from build123d import *

# Parameters (mm, degrees)
F0_W       = 85
F0_H       = 85
F1_DEPTH   = 3
F2_W       = 13.4
F2_H       = 13.4
F3_DEPTH   = 25
F5_DEPTH   = 15
F6_SIZE2   = 14.99999
F6_SIZE    = 9.99999
F6_2_SIZE2 = 14.99999
F6_2_SIZE  = 9.99999
F6_3_SIZE2 = 14.99999
F6_3_SIZE  = 9.99999
F6_4_SIZE2 = 14.99999
F6_4_SIZE  = 9.99999
F7_SIZE2   = 9.99999
F7_SIZE    = 14.99999
F7_2_SIZE2 = 9.99999
F7_2_SIZE  = 14.99999
F7_3_SIZE2 = 9.99999
F7_3_SIZE  = 14.99999
F7_4_SIZE2 = 9.99999
F7_4_SIZE  = 14.99999
F7_5_SIZE2 = 9.99999
F7_5_SIZE  = 14.99999
F9_DEPTH   = 68.601
F11_DEPTH  = 68.601


# Not quite as in the source:
# - a fillet or chamfer is up to 0.001 mm smaller than in the source, because OpenCascade refuses the exact size
# - a feature names something its author has since deleted; it is built from what else it names


with BuildPart() as f1:
    # F0 (on Top) → F1 (new body)
    with BuildSketch(Plane.XY):
        Rectangle(F0_W, F0_H)
    extrude(amount=F1_DEPTH)

    # F2 (on face) → F3 (cut)
    with BuildSketch(Plane.XY.offset(3)):
        with Locations((-32.8, 16.4)):
            Rectangle(F2_W, F2_H)
        with Locations((-32.8, 0)):
            Rectangle(F2_W, F2_H)
        with Locations((-32.8, -16.4)):
            Rectangle(F2_W, F2_H)
        with Locations((-32.8, -32.8)):
            Rectangle(F2_W, F2_H)
        with Locations((-16.4, 32.8)):
            Rectangle(F2_W, F2_H)
        with Locations((-16.4, 16.4)):
            Rectangle(F2_W, F2_H)
        with Locations((-16.4, 0)):
            Rectangle(F2_W, F2_H)
        with Locations((-16.4, -16.4)):
            Rectangle(F2_W, F2_H)
        with Locations((-16.4, -32.8)):
            Rectangle(F2_W, F2_H)
        with Locations((0, 32.8)):
            Rectangle(F2_W, F2_H)
        with Locations((0, 16.4)):
            Rectangle(F2_W, F2_H)
        Rectangle(F2_W, F2_H)
        with Locations((0, -16.4)):
            Rectangle(F2_W, F2_H)
        with Locations((0, -32.8)):
            Rectangle(F2_W, F2_H)
        with Locations((16.4, 32.8)):
            Rectangle(F2_W, F2_H)
        with Locations((16.4, 16.4)):
            Rectangle(F2_W, F2_H)
        with Locations((16.4, 0)):
            Rectangle(F2_W, F2_H)
        with Locations((16.4, -16.4)):
            Rectangle(F2_W, F2_H)
        with Locations((16.4, -32.8)):
            Rectangle(F2_W, F2_H)
        with Locations((32.8, 32.8)):
            Rectangle(F2_W, F2_H)
        with Locations((32.8, 16.4)):
            Rectangle(F2_W, F2_H)
        with Locations((32.8, 0)):
            Rectangle(F2_W, F2_H)
        with Locations((32.8, -16.4)):
            Rectangle(F2_W, F2_H)
        with Locations((32.8, -32.8)):
            Rectangle(F2_W, F2_H)
        with Locations((-32.8, 32.8)):
            Rectangle(F2_W, F2_H)
    extrude(amount=-F3_DEPTH, mode=Mode.SUBTRACT)

    # F4 (on face) → F5 (join)
    with BuildSketch(Plane.XY.offset(3)):
        Polygon((-23.1, -9.7), (-26.1, -9.7), (-26.1, -23.1), (-39.5, -23.1), (-39.5, -26.1), (-26.1, -26.1), (-26.1, -39.5), (-23.1, -39.5), (-23.1, -26.1), (-9.7, -26.1), (-9.7, -23.1), (-23.1, -23.1), align=None)
        Polygon((-9.7, 23.1), (-9.7, 26.1), (-23.1, 26.1), (-23.1, 39.5), (-26.1, 39.5), (-26.1, 26.1), (-39.5, 26.1), (-39.5, 23.1), (-26.1, 23.1), (-26.1, 9.7), (-23.1, 9.7), (-23.1, 23.1), align=None)
        Polygon((26.1, 26.1), (26.1, 39.5), (23.1, 39.5), (23.1, 26.1), (9.7, 26.1), (9.7, 23.1), (23.1, 23.1), (23.1, 9.7), (26.1, 9.7), (26.1, 23.1), (39.5, 23.1), (39.5, 26.1), align=None)
        Polygon((26.1, -23.1), (26.1, -9.7), (23.1, -9.7), (23.1, -23.1), (9.7, -23.1), (9.7, -26.1), (23.1, -26.1), (23.1, -39.5), (26.1, -39.5), (26.1, -26.1), (39.5, -26.1), (39.5, -23.1), align=None)
    extrude(amount=F5_DEPTH)

    # F6 (size 10 and 15 in the source; OpenCascade refuses exactly that, so slightly less here)
    f6_edges = [f1.edges().sort_by_distance(p)[0] for p in [
        (-39.5, -24.6, 18),
        (-24.6, -9.7, 18),
        (-9.7, -24.6, 18),
        (-24.6, -39.5, 18),
    ]]
    f6_side = f1.faces().sort_by_distance((-24.6, -24.6, 18))[0]
    chamfer(f6_edges, length=F6_SIZE, length2=F6_SIZE2, reference=f6_side)

    # F6#2 (size 10 and 15 in the source; OpenCascade refuses exactly that, so slightly less here)
    f6_2_edges = [f1.edges().sort_by_distance(p)[0] for p in [
        (-39.5, 24.6, 18),
        (-24.6, 39.5, 18),
    ]]
    f6_2_side = f1.faces().sort_by_distance((-24.6, 24.6, 18))[0]
    chamfer(f6_2_edges, length=F6_2_SIZE, length2=F6_2_SIZE2, reference=f6_2_side)

    # F6#3 (size 10 and 15 in the source; OpenCascade refuses exactly that, so slightly less here)
    f6_3_edges = [f1.edges().sort_by_distance(p)[0] for p in [
        (9.7, 24.6, 18),
        (24.6, 39.5, 18),
    ]]
    f6_3_side = f1.faces().sort_by_distance((24.6, 24.6, 18))[0]
    chamfer(f6_3_edges, length=F6_3_SIZE, length2=F6_3_SIZE2, reference=f6_3_side)

    # F6#4 (size 10 and 15 in the source; OpenCascade refuses exactly that, so slightly less here)
    f6_4_edges = [f1.edges().sort_by_distance(p)[0] for p in [
        (24.6, -9.7, 18),
        (9.7, -24.6, 18),
        (39.5, -24.6, 18),
    ]]
    f6_4_side = f1.faces().sort_by_distance((24.6, -24.6, 18))[0]
    chamfer(f6_4_edges, length=F6_4_SIZE, length2=F6_4_SIZE2, reference=f6_4_side)

    # F7 (size 15 and 10 in the source; OpenCascade refuses exactly that, so slightly less here)
    f7_edges = [f1.edges().sort_by_distance(p)[0] for p in [
        (-9.7, 24.6, 18),
    ]]
    f7_side = f1.faces().sort_by_distance((-9.7, 24.6, 10.5))[0]
    chamfer(f7_edges, length=F7_SIZE, length2=F7_SIZE2, reference=f7_side)

    # F7#2 (size 15 and 10 in the source; OpenCascade refuses exactly that, so slightly less here)
    f7_2_edges = [f1.edges().sort_by_distance(p)[0] for p in [
        (-24.6, 9.7, 18),
    ]]
    f7_2_side = f1.faces().sort_by_distance((-24.6, 9.7, 10.5))[0]
    chamfer(f7_2_edges, length=F7_2_SIZE, length2=F7_2_SIZE2, reference=f7_2_side)

    # F7#3 (size 15 and 10 in the source; OpenCascade refuses exactly that, so slightly less here)
    f7_3_edges = [f1.edges().sort_by_distance(p)[0] for p in [
        (24.6, 9.7, 18),
    ]]
    f7_3_side = f1.faces().sort_by_distance((24.6, 9.7, 10.5))[0]
    chamfer(f7_3_edges, length=F7_3_SIZE, length2=F7_3_SIZE2, reference=f7_3_side)

    # F7#4 (size 15 and 10 in the source; OpenCascade refuses exactly that, so slightly less here)
    f7_4_edges = [f1.edges().sort_by_distance(p)[0] for p in [
        (39.5, 24.6, 18),
    ]]
    f7_4_side = f1.faces().sort_by_distance((39.5, 24.6, 10.5))[0]
    chamfer(f7_4_edges, length=F7_4_SIZE, length2=F7_4_SIZE2, reference=f7_4_side)

    # F7#5 (size 15 and 10 in the source; OpenCascade refuses exactly that, so slightly less here)
    f7_5_edges = [f1.edges().sort_by_distance(p)[0] for p in [
        (24.6, -39.5, 18),
    ]]
    f7_5_side = f1.faces().sort_by_distance((24.6, -39.5, 10.5))[0]
    chamfer(f7_5_edges, length=F7_5_SIZE, length2=F7_5_SIZE2, reference=f7_5_side)

    # F8 (on face) → F9 (cut, through all)
    with BuildSketch(Plane.YZ.offset(26.1)):
        Polygon((-26.1, 17), (-26.5611153912, 17), (-35.8944487245, 3), (-26.1, 3), align=None)
        Polygon((-22.6388846088, 17), (-23.1, 17), (-23.1, 3), (-13.3055512755, 3), align=None)
        Polygon((23.1, 17), (22.6388846088, 17), (13.3055512755, 3), (23.1, 3), align=None)
        Polygon((26.5611153912, 17), (26.1, 17), (26.1, 3), (35.8944487245, 3), align=None)
    extrude(amount=-F9_DEPTH, mode=Mode.SUBTRACT)

    # F10 (on face) → F11 (cut, through all)
    with BuildSketch(Plane.XZ.offset(26.1)):
        Polygon((-26.1, 17), (-26.5611153912, 17), (-35.8944487245, 3), (-26.1, 3), align=None)
        Polygon((-22.6388846088, 17), (-23.1, 17), (-23.1, 3), (-13.3055512755, 3), align=None)
        Polygon((23.1, 17), (22.6388846088, 17), (13.3055512755, 3), (23.1, 3), align=None)
        Polygon((26.5611153912, 17), (26.1, 17), (26.1, 3), (35.8944487245, 3), align=None)
    extrude(amount=-F11_DEPTH, mode=Mode.SUBTRACT)


solid = f1.part
CAD build for the part. Positions are in the model's coordinates, mm. A direction names the side the tool comes from. Round coordinates to 2 decimals unless told otherwise and drop trailing zeros. Order: outer loops, then holes, each group sorted by start corner. A loop starts at its lowest first (then second) coordinate and runs counter-clockwise, first axis right, second up. Notation, with made-up numbers: (52.25, 5) -> (79.25, 5) arc R31 cw to (79.25, 32) -> close; hole circle Ø6 at (-38.75, 49.25). An arc over 180 degrees is marked (long way). Write item = value, one per line. Start each with the question number.
(1) Pin check, flat tips, straight feed: P1, Ø6.5, axis at y = 33, z = 12.5, coming from the -X side; P2, Ø2, axis at y = -33.5, z = 5.5, coming from the +X side; P3, Ø1, axis at x = 12, y = 21.5, coming from the -Z side; P4, Ø0.5, axis at x = -26.5, y = -24.5, coming from the -Z side. Stop position of each tip, or through.
(2) Cut at A-A, the plane y = -2.5. List the corners of the cut face in (x, z).
(3) Pull direction Y, two halves, no side cores. Call faces 5 (the flat face through (-23.1, 15, 7)), 6 (the flat face through (-26.1, 25, 10)): released by +Y, released by -Y, zero draft, split by the parting line, or undercut.
(4) Probe line 1 (Y direction, x = 19, z = 1.75); line 2 (Y direction, x = 38, z = 4.5). List the from-to ranges inside material, lowest first. Write a range as [from, to].
(5) Which spindle directions (+Z, -Z, +X, -X, +Y, -Y) get a long thin tool onto all of the face, cutting with end or side? Do faces 1 (the flat face through (-24.621, 14.77, 10.605)), 2 (the flat face through (33, 9.7, 2)), 3 (the flat face through (-25, -18, 3)), 4 (the flat face through (-18, 25, 3)). Say none if no direction does.
(6) Cut at B-B, the plane y = -31.5. State how many separate pieces and enclosed holes the cut face has, then the cut area to 4 significant figures.
Model answer:
q1.P1 = -26.1
q1.P2 = 26.1
q1.P3 = through
q1.P4 = 0
q2.outline = (-42.5, 0) -> (-39.5, 0) -> (-39.5, 3) -> (-42.5, 3) -> close; (-26.1, 0) -> (-23.1, 0) -> (-23.1, 3) -> (-26.1, 3) -> close; (-9.7, 0) -> (-6.7, 0) -> (-6.7, 3) -> (-9.7, 3) -> close; (6.7, 0) -> (9.7, 0) -> (9.7, 3) -> (6.7, 3) -> close; (23.1, 0) -> (26.1, 0) -> (26.1, 3) -> (23.1, 3) -> close; (39.5, 0) -> (42.5, 0) -> (42.5, 3) -> (39.5, 3) -> close
q3.face_5 = undercut
q3.face_6 = zero draft
q4.line_1 = [-42.5, -39.5], [-26.1, -23.1], [-9.7, -6.7], [6.7, 9.7], [23.1, 26.1], [39.5, 42.5]
q4.line_2 = [-26.1, -23.1], [23.1, 26.1]
q5.face_1 = +Z, +X, -X
q5.face_2 = +Z, -Z
q5.face_3 = +X, -X
q5.face_4 = +Y, -Y
q6.separate_pieces = 8
q6.enclosed_holes = 0
q6.area = 86.45 mm2
